Geometry: final body of the model. Coordinates: model frame, mm. A direction names the side the tool comes from. Coordinates: 2 decimals unless noted, no trailing zeros. Loops run counter-clockwise (first coordinate to the right, second up) from the corner with the lowest first, then second, coordinate; pieces in that order, holes last. Notation, with made-up numbers: (25, 14.5) - (47, 14.5) arc R21 cw to (47, 41.5) - close; hole circle Ø8 at (-11.5, -35.75). An arc over 180 degrees is marked (long way). Put each result on its own line as item: value. Start each with the question number.
1) Draft query along Z for faces 1 (the flat face through (0, 153, -49)), 2 (the conical face through (29.38, 14.56, -290.58)), 3 (the flat face through (128, 153, -310)). Return one class per face: +Z half, -Z half, draft (parallel to the pull), parting line (faces both ways), or undercut.
2) Reachability of faces 4 (the cylindrical face through (255.07, 166.26, -190.77)), 5 (the cylindrical face through (13.8, 11.5, -17.7)) from +Z, -Z, +X, -X, +Y, -Y: full face, straight path, thin tool, end or side. Return the list, or none.
3) Section C-C on z = -226.5. Output: boundary loops of the cut face in (x, y), and give its area (3 significant figures).
4) Section D-D on y = 67. Output: boundary loops of the cut face in (x, z), and give its area (3 significant figures).
5) Section A-A on x = 70. Output: boundary loops of the cut face in (y, z), and give its area (3 significant figures).
6) Material intervals for line 1 along Z through (x, y) = (19, 295); line 2 along Y through (x, z) = (12, -290); line 3 along X through (y, z) = (231.5, -203), sorted ascending. Write a range as from..to.
7) Section B-B on y = 155. Output: boundary loops of the cut face in (x, z).
8) Contact query for flat-ended pins moving along their axis: pin 1 Ø5 at (y, z) = (295, -20) entering from -X; pin 2 Ø5 at (y, z) = (249.5, -184.5) entering from -X. Output: stop coordinate, or through.
Autodesk Inventor part; units mm, degrees
ref_plane "YZ Plane" through (0, 0, 0) normal (1, 0, 0) x (0, 1, 0)
ref_plane "XZ Plane" through (0, 0, 0) normal (0, 1, 0) x (-1, 0, 0)
ref_plane "XY Plane" through (0, 0, 0) normal (0, 0, 1) x (1, 0, 0)
sketch "Skizze1" plane through (0, 0, 0) normal (1, 0, 0) x (0, 1, 0)
  line L0 (0, 0) -> (310, 0)
  line L1 (310, 0) -> (310, -310)
  line L2 (310, -310) -> (0, -310)
  line L3 (0, -310) -> (0, 0)
  dimension "d0" = 310
  dimension "d1" = 310
sketch "Skizze2" plane through (0, 0, 0) normal (1, 0, 0) x (0, 1, 0)
  circle A0 centre (155, -155) radius 105
  point P0 (0, 0)
  dimension "d4" = 210
extrude "Extrusion1" add sketch "Skizze1" along normal blind 250
extrude "Extrusion2" cut sketch "Skizze2" along normal blind 250
sketch "Skizze3" plane through (250, 0, 0) normal (1, 0, 0) x (0, 0, -1)
  line L0 (0, 310) -> (0, 0)
  line L1 (310, 310) -> (0, 310)
  line L2 (0, 0) -> (310, 0)
  line L3 (310, 0) -> (310, 310)
  line L4 (310, 310) -> (0, 310)
  line L5 (0, 310) -> (0, 0)
extrude "Extrusion3" add sketch "Skizze3" along normal blind 10
sketch "Skizze4" plane through (260, 0, 0) normal (1, 0, 0) x (0, 0, -1)
  circle A0 centre (155, 155) radius 37.5
  point P0 (0, 0)
  dimension "d13" = 75
extrude "Extrusion4" cut sketch "Skizze4" against normal blind 10
sketch "Skizze5" plane through (0, 0, 0) normal (-1, 0, 0) x (0, 0, 1)
  line L0 (-310, 0) -> (-310, 310)
  line L1 (-310, 310) -> (-290, 310)
  line L2 (-290, 310) -> (-290, 295)
  line L3 (-290, 295) -> (-310, 295)
  line L4 (-310, 295) -> (-310, 310)
  line L5 (-310, 310) -> (0, 310)
  line L6 (0, 310) -> (-20, 310)
  line L7 (-20, 310) -> (-20, 295)
  line L8 (-20, 295) -> (0, 295)
  line L9 (0, 295) -> (0, 310)
  line L10 (0, 0) -> (-310, 0)
  line L11 (0, 0) -> (-20, 0)
  line L12 (-20, 0) -> (-20, 15)
  line L13 (-20, 15) -> (0, 15)
  line L14 (0, 15) -> (0, 0)
  line L15 (-310, 0) -> (-290, 0)
  line L16 (-290, 0) -> (-290, 15)
  line L17 (-290, 15) -> (-310, 15)
  line L18 (-310, 15) -> (-310, 0)
  dimension "d16" = 20
  dimension "d17" = 15
  dimension "d18" = 20
  dimension "d19" = 15
hole "Bohrung1" at (0, 295, -290) at (0, 295, -20) at (0, 15, -20) at (0, 15, -290) direction (1, 0, 0) diameter 8.376 depth 27.3 tip angle 118
properties part number "Führung_hochfahren"
Answer block:
1. face 1: draft
1. face 2: undercut
1. face 3: -Z half
2. face 4: +X, -X
2. face 5: -X
3. outline: (0, 0) - (260, 0) - (260, 310) - (0, 310) - (0, 231.89) - (250, 231.89) - (250, 78.11) - (0, 78.11) - close
3. area: 42,200 mm²
4. outline: (0, -310) - (260, -310) - (260, 0) - (0, 0) - (0, -97.72) - (250, -97.72) - (250, -212.28) - (0, -212.28) - close
4. area: 52,000 mm²
5. outline: (0, -310) - (310, -310) - (310, 0) - (0, 0) - close; hole circle Ø210 at (155, -155)
5. area: 61,500 mm²
6. line 1: z = -310..-294.19, -285.81..-24.19, -15.81..0
6. line 2: y = 0..10.81, 19.19..290.81, 299.19..310
6. line 3: x = 250..260
7. outline: (0, -310) - (260, -310) - (260, -192.5) - (250, -192.5) - (250, -260) - (0, -260) - close; (0, -50) - (250, -50) - (250, -117.5) - (260, -117.5) - (260, 0) - (0, 0) - close
8. pin 1: stops at x = 28.31
8. pin 2: stops at x = 250
